The model under review builds one solid part; all positions refer to its coordinate system, in mm. A direction names the side the tool comes from. Round coordinates to 2 decimals unless told otherwise and drop trailing zeros. One line per question, with ' | ' between items.
from build123d import *

# Parameters (mm, degrees)
SKETCH1_W                                            = 12
SKETCH1_H                                            = 2.9
CBORE_FOR_M2_5_HEX_SOCKET_HEAD_CAP_SCREW_D           = 2.9
CBORE_FOR_M2_5_HEX_SOCKET_HEAD_CAP_SCREW_CBORE_D     = 5.5
CBORE_FOR_M2_5_HEX_SOCKET_HEAD_CAP_SCREW_CBORE_DEPTH = 2.1
CIRPATTERN1_COUNT                                    = 6
CUT_EXTRUDE4_DEPTH                                   = 3.9
SKETCH5_R                                            = 24.475
SKETCH5_R_2                                          = 18.8
BOSS_EXTRUDE1_DEPTH                                  = 1


with BuildPart() as part:
    # Sketch1 → Revolve1 (revolve)
    with BuildSketch(Plane.XY):
        with Locations((-18.5, 1.45)):
            Rectangle(SKETCH1_W, SKETCH1_H)
    revolve(axis=Axis((0, -3.243860323, 0), (0, 1, 0)))

    # CBORE for M2.5 Hex Socket Head Cap Screw2 (through all)
    with Locations(Plane(origin=(0, 3.4, 0), x_dir=(-1, 0, 0), z_dir=(0, 1, 0))):
        with Locations((0, -15.5)):
            cbore_for_m2_5_hex_socket_head_cap_screw = CounterBoreHole(CBORE_FOR_M2_5_HEX_SOCKET_HEAD_CAP_SCREW_D / 2, CBORE_FOR_M2_5_HEX_SOCKET_HEAD_CAP_SCREW_CBORE_D / 2, CBORE_FOR_M2_5_HEX_SOCKET_HEAD_CAP_SCREW_CBORE_DEPTH)

    # CirPattern1: CBORE for M2.5 Hex Socket Head Cap Screw2 ×6 about axis
    cirpattern1_axis = Axis((0, 0, 0), (0, 1, 0))
    for i in range(1, CIRPATTERN1_COUNT):
        add(cbore_for_m2_5_hex_socket_head_cap_screw.rotate(cirpattern1_axis, i * 360 / CIRPATTERN1_COUNT), mode=Mode.SUBTRACT)

    # Sketch10 → Cut-Extrude4 (cut, through all)
    with BuildSketch(Plane(origin=(0, 2.9, 0), x_dir=(1, 0, 0), z_dir=(0, 1, 0))):
        with BuildLine():
            Line((-15, -1.5), (-17, -1.5))
            ThreePointArc((-17, -1.5), (-18.5, 0), (-17, 1.5))
            Line((-17, 1.5), (-15, 1.5))
            ThreePointArc((-15, 1.5), (-13.5, 0), (-15, -1.5))
        make_face()
    extrude(amount=-CUT_EXTRUDE4_DEPTH, mode=Mode.SUBTRACT)

    # Sketch5 → Boss-Extrude1 (add)
    with BuildSketch(Plane(origin=(0, 2.9, 0), x_dir=(1, 0, 0), z_dir=(0, 1, 0))):
        Circle(SKETCH5_R)
        Circle(SKETCH5_R_2, mode=Mode.SUBTRACT)
    extrude(amount=BOSS_EXTRUDE1_DEPTH)


solid = part.part
1) Mouldability with a two-part tool opening along Z and no side actions: class faces 3 (the cylindrical face through (-13.17, 1.47, 20.66)), 4 (the flat face through (-16, 1, -1.5)), 5 (the flat face through (-6, 3.9, 18)) as +Z half, -Z half, draft (parallel to the pull), parting line (faces both ways), or undercut.
Output values:
face 3: parting line | face 4: undercut | face 5: draft
2) Insertion check: P1, Ø6.5, axis at x = -13.42, z = -7.75, coming from the +Y side; P2, Ø3.5, axis at x = 0, z = 15.5, coming from the -Y side; P3, Ø0.6, axis at x = -16, y = 1, coming from the -Z side; P4, Ø2, axis at x = -6.5, z = 7, coming from the -Y side. Each pin has a flat end and moves straight along its axis. Give the tip position at first contact, or say it passes through.
Output values:
P1: stops at y = 2.9 | P2: stops at y = 0 | P3: stops at z = -18.81 | P4: passes through
3) Add section A-A on x = 0. State how many separate pieces and enclosed holes the cut face has, then the cut area to 3 significant figures.
Output values:
separate pieces: 4 | enclosed holes: 0 | area: 55.8 mm²
4) For line 1 (Z direction, x = 0, y = 1.9); line 2 (Z direction, x = 0, y = 0.6); line 3 (Z direction, x = -10.5, y = 3.15), list the stretches that pass through material, from the lowest coordinate up.
Output values:
line 1: z = -24.5 to -18.25, -12.75 to -12.5, 12.5 to 12.75, 18.25 to 24.5 | line 2: z = -24.5 to -16.95, -14.05 to -12.5, 12.5 to 14.05, 16.95 to 24.5 | line 3: z = -22.11 to -15.59, 15.59 to 22.11
5) Machinability: for faces 1 (the flat face through (-16, 1, 1.5)), 2 (the cylindrical face through (-4.08, 3.39, 18.35)), which of the approach directions +Z, -Z, +X, -X, +Y, -Y give a long, thin tool a straight path to every point of the face, cutting with its end or side? Answer none if there is none.
Output values:
face 1: +Y, -Y | face 2: +Y
